from build123d import *

# Parameters (mm, degrees)
SKETCH2_W           = 292.1
SKETCH2_H           = 292.1
BOSS_EXTRUDE1_DEPTH = 146.05
SHELL1_T            = -12.7
SKETCH3_W           = 44.121317042
SKETCH3_H           = 266.7
CUT_EXTRUDE1_DEPTH  = 12.7
SKETCH4_W           = 8.89
SKETCH4_H           = 10.922
CUT_EXTRUDE2_DEPTH  = 2.54


with BuildPart() as part:
    # Sketch2 → Boss-Extrude1 (new body, symmetric)
    with BuildSketch(Plane.XY):
        Rectangle(SKETCH2_W, SKETCH2_H)
    extrude(amount=BOSS_EXTRUDE1_DEPTH, both=True)

    # Shell1
    shell1_openings = [part.faces().sort_by_distance(p)[0] for p in [
        (0, 0, 146.05),
    ]]
    offset(amount=SHELL1_T, openings=shell1_openings, kind=Kind.INTERSECTION)

    # Sketch3 → Cut-Extrude1 (cut)
    with BuildSketch(Plane.XY.offset(146.05)):
        with Locations((-133.35, 0)):
            Rectangle(SKETCH3_W, SKETCH3_H)
    extrude(amount=-CUT_EXTRUDE1_DEPTH, mode=Mode.SUBTRACT)

    # Sketch4 → Cut-Extrude2 (cut)
    with BuildSketch(Plane(origin=(0, 0, -146.05), x_dir=(-1, 0, 0), z_dir=(0, 0, -1))):
        with Locations((-90.805, -89.789)):
            Rectangle(SKETCH4_W, SKETCH4_H)
    extrude(amount=-CUT_EXTRUDE2_DEPTH, mode=Mode.SUBTRACT)


solid = part.part
Source: CAD feature listing. Evaluate the final solid. Frame: model axes, mm. A direction names the side the tool comes from. Round coordinates to 2 decimals unless told otherwise and drop trailing zeros. Loops run counter-clockwise (first coordinate to the right, second up) from the corner with the lowest first, then second, coordinate; pieces in that order, holes last. Notation, with made-up numbers: (69, -8.5) - (87, -8.5) arc R16 ccw to (87, 13.5) - close; hole circle Ø3 at (78, -32). An arc over 180 degrees is marked (long way). Write item = value, one per line. Start each with the question number.
(1) Ray query, line 1 along Y through (x, z) = (56.5, 36); line 2 along Z through (x, y) = (107, 80). Return the intervals inside material, ascending. Write a range as from..to.
(2) Pull-direction query (Y, two-part tool) for faces 1 (the face through (140, 1, 146.05)), 2 (the face through (-8, -133.35, 8)), 3 (the face through (-2, 146.05, 2)); classes: +Y half, -Y half, draft (parallel to the pull), parting line (faces both ways), or undercut.
(3) Section query C-C, the plane x = -31.5. Output: boundary loops of the cut face in (y, z).
(4) Section query A-A, the plane z = -109.5. Output: boundary loops of the cut face in (x, y), plus the area to 3 significant figures.
(5) Section query B-B, the plane y = 103. Output: boundary loops of the cut face in (x, z), plus the area to 3 significant figures.
(6) Set-up query: faces 4 (the face through (-140, 2, 133.35)), 5 (the face through (133.35, -2, 8)), 6 (the face through (91, -90, -143.51)), 7 (the face through (-2, -146.05, 2)). Return all of +Z, -Z, +X, -X, +Y, -Y with unobstructed straight access to the full face (end or side cutting, diameter ignored); none if empty.
(7) Pin query (flat end, axial travel): pin 1 (4.5 mm diameter, centred on x = 89, y = -87.5, fed in from -Z); pin 2 (4 mm diameter, centred on x = -140.5, y = -22, fed in from +Z). Return the tip coordinate at first contact, or that it passes through.
Conclusion:
q1.line_1 = -146.05..-133.35, 133.35..146.05
q1.line_2 = -146.05..-133.35
q2.face_1 = draft
q2.face_2 = undercut
q2.face_3 = +Y half
q3.outline = (-146.05, -146.05) - (146.05, -146.05) - (146.05, 146.05) - (133.35, 146.05) - (133.35, -133.35) - (-133.35, -133.35) - (-133.35, 146.05) - (-146.05, 146.05) - close
q4.outline = (-146.05, -146.05) - (146.05, -146.05) - (146.05, 146.05) - (-146.05, 146.05) - close; hole (-133.35, -133.35) - (133.35, -133.35) - (133.35, 133.35) - (-133.35, 133.35) - close
q4.area = 14,200 mm2
q5.outline = (-146.05, -146.05) - (146.05, -146.05) - (146.05, 146.05) - (133.35, 146.05) - (133.35, -133.35) - (-133.35, -133.35) - (-133.35, 133.35) - (-146.05, 133.35) - close
q5.area = 10,600 mm2
q6.face_4 = +Z, -X
q6.face_5 = +Z
q6.face_6 = -Z
q6.face_7 = +Z, -Z, +X, -X, -Y
q7.pin_1 = -143.51
q7.pin_2 = 133.35
